```python
from build123d import *

# Parameters (mm, degrees)
SKETCH004_R             = 52
SKETCH004_R_2           = 2
SKETCH004_R_3           = 1.8
PAD003_DEPTH            = 3
SKETCH006_R             = 1.8
POCKET001_DEPTH         = 0.001
POCKET001_DEPTH_BACK    = 3.001
BODY002_PLACEMENT_ANGLE = 180


with BuildPart() as part:
    # Sketch004 → Pad003 (new body)
    with BuildSketch(Plane.XY):
        Circle(SKETCH004_R)
        Circle(SKETCH004_R_2, mode=Mode.SUBTRACT)
        with Locations((8.485281, 8.485281)):
            Circle(SKETCH004_R_3, mode=Mode.SUBTRACT)
        with Locations((-8.485281, 8.485281)):
            Circle(SKETCH004_R_3, mode=Mode.SUBTRACT)
        with Locations((-8.485281, -8.485281)):
            Circle(SKETCH004_R_3, mode=Mode.SUBTRACT)
        with Locations((8.485281, -8.485281)):
            Circle(SKETCH004_R_3, mode=Mode.SUBTRACT)
    extrude(amount=PAD003_DEPTH)

    # Sketch006 → Pocket001 (cut, two sides)
    with BuildSketch(Plane.XY) as pocket001_sk:
        with Locations((-33.234019, 33.234019)):
            Circle(SKETCH006_R)
        with Locations((-33.234019, -33.234019)):
            Circle(SKETCH006_R)
        with Locations((33.234019, -33.234019)):
            Circle(SKETCH006_R)
        with Locations((33.234019, 33.234019)):
            Circle(SKETCH006_R)
    extrude(amount=-POCKET001_DEPTH, mode=Mode.SUBTRACT)
    extrude(pocket001_sk.sketch, amount=POCKET001_DEPTH_BACK, mode=Mode.SUBTRACT)

    # Sphere → Sphere (revolve)
    with BuildSketch(Plane.XZ.offset(-47)):
        with BuildLine():
            ThreePointArc((5, 0), (3.535534, 3.535534), (0, 5))
            Line((0, 5), (0, 0))
            Line((0, 0), (5, 0))
        make_face()
    revolve(axis=Axis((0, 47, 0), (0, 0, 1)))

    # Sphere001 → Sphere001 (revolve)
    with BuildSketch(Plane.XZ.offset(47)):
        with BuildLine():
            ThreePointArc((5, 0), (3.535534, 3.535534), (0, 5))
            Line((0, 5), (0, 0))
            Line((0, 0), (5, 0))
        make_face()
    revolve(axis=Axis((0, -47, 0), (0, 0, 1)))

    # Sphere002 → Sphere002 (revolve)
    with BuildSketch(Plane(origin=(47, 0, 0), x_dir=(1, 0, 0), z_dir=(0, -1, 0))):
        with BuildLine():
            ThreePointArc((5, 0), (3.535534, 3.535534), (0, 5))
            Line((0, 5), (0, 0))
            Line((0, 0), (5, 0))
        make_face()
    revolve(axis=Axis((47, 0, 0), (0, 0, 1)))

    # Sphere003 → Sphere003 (revolve)
    with BuildSketch(Plane(origin=(-47, 0, 0), x_dir=(1, 0, 0), z_dir=(0, -1, 0))):
        with BuildLine():
            ThreePointArc((5, 0), (3.535534, 3.535534), (0, 5))
            Line((0, 5), (0, 0))
            Line((0, 0), (5, 0))
        make_face()
    revolve(axis=Axis((-47, 0, 0), (0, 0, 1)))


with BuildPart() as part_1:
    # Body002 placement: moved
    add(part.part.moved(Location((0, 0, 53))).rotate(Axis((0, 0, 53), (0, 0, -1)), BODY002_PLACEMENT_ANGLE))


solid = part_1.part
```
Geometry check sheet. Reference: the model listing, model coordinates, mm. A direction names the side the tool comes from. Round coordinates to 2 decimals unless told otherwise and drop trailing zeros. Write each loop counter-clockwise with the first axis right and the second up, starting at its lowest first coordinate (ties: lowest second). Pieces come first, ordered by that corner, then holes. Notation, with made-up numbers: (80.25, 10.5) -> (93.25, 10.5) arc R14 ccw to (93.25, 31.5) -> close; hole circle Ø11 at (4, 30). An arc over 180 degrees is marked (long way). Put each result on its own line as item: value.
1) Access from +Z, -Z, +X, -X, +Y, -Y to the whole of each face (thin tool, end or side, straight path). Record for faces 5 (the face through (-11, -1, 56)), 6 (the face through (8.88, 10.24, 54.48)).
Recorded:
face 5: +Z
face 6: +Z, -Z
2) Release check for a two-part mould opening along X. For faces 1 (the face through (-10.2, -9.03, 54.48)), 2 (the face through (32.4, 34.83, 54.48)), 3 (the face through (-11, -1, 53)), 4 (the face through (41.265, 31.641, 54.479)) record: pulls with the +X half, pulls with the -X half, needs draft (parallel to the pull), parting line crosses it, or undercut.
Recorded:
face 1: undercut
face 2: undercut
face 3: needs draft
face 4: parting line crosses it
3) Thickness scan on probe 1 along Y at (x, z) = (0, 54.9); probe 2 along Z at (x, y) = (19, 21); probe 3 along Y at (x, z) = (9.5, 53.55). Record the ranges inside material, lowest first. Write a range as from..to.
Recorded:
probe 1: y = -52..-2, 2..52
probe 2: z = 53..56
probe 3: y = -51.12..-9.97, -7..7, 9.97..51.12
4) Cross-section at D-D, the plane x = -25. Enter the section's corners in (y, z), plus the area to 3 significant figures.
Recorded:
outline: (-45.6, 53) -> (45.6, 53) -> (45.6, 56) -> (-45.6, 56) -> close
area: 274 mm2
5) Cross-section at B-B, the plane z = 54.05. Give the number of separate pieces and of enclosed holes in the cut face, plus the area to 3 significant figures.
Recorded:
separate pieces: 1
enclosed holes: 9
area: 8,400 mm2
6) Cross-section at A-A, the plane x = 8.5. Enter the section's corners in (y, z), plus the area to 3 significant figures.
Recorded:
outline: (-51.3, 53) -> (-10.29, 53) -> (-10.29, 56) -> (-51.3, 56) -> close; (-6.69, 53) -> (6.69, 53) -> (6.69, 56) -> (-6.69, 56) -> close; (10.29, 53) -> (51.3, 53) -> (51.3, 56) -> (10.29, 56) -> close
area: 286 mm2
7) Cross-section at C-C, the plane y = 29.5. Enter the section's corners in (x, z).
Recorded:
outline: (-42.82, 53) -> (42.82, 53) -> (42.82, 56) -> (-42.82, 56) -> close
8) Depth check by flat-ended pin: P1, Ø4.5, axis at x = 33.23, y = -33.23, coming from the +Z side; P2, Ø1, axis at y = 15, z = 56, coming from the +X side; P3, Ø2, axis at x = 5.5, z = 55, coming from the -Y side. Enter the tip coordinate at first touch or a pass-through.
Recorded:
P1: stops at z = 56
P2: stops at x = 49.94
P3: stops at y = -51.8
